Answer from the drawing. Dimensions are ordinates in mm from the lowest x, y and z of the part. A direction names the side the tool comes from. Round coordinates to 2 decimals unless told otherwise and drop trailing zeros. Order: outer loops, then holes, each group sorted by start corner. A loop starts at its lowest first (then second) coordinate and runs counter-clockwise, first axis right, second up. Notation, with made-up numbers: (54.5, 29.25) - (66.5, 29.25) arc R34 ccw to (66.5, 68.25) - close; hole circle Ø10 at (86, 47.5). An arc over 180 degrees is marked (long way). One line per question, with ' | ' between items. Start each with the question number.
1) For the marked faces 1 and 2, determine the directions among +Z, -Z, +X, -X, +Y, -Y from which every point of the face is accessible in a straight line to the end or side of a thin tool.
2) The part is cut by section D-D, the plane z = 1.35. Give the vertices of the cut face in (x, y).
3) Straight lines are drawn through the part: line 1 (Y direction, x = 6.5, z = 0.05); line 2 (Z direction, x = 4, y = 9.5); line 3 (Y direction, x = 5, z = 1.75) (1 decimal). For each, find the intervals that lie inside material, in ascending order. Write a range as from..to.
4) Flat-ended cylindrical pins translate along their axes: pin 1 (1 mm diameter, centred on y = 8, z = 2.5, fed in from +X); pin 2 (4 mm diameter, centred on x = 7.5, y = 8, fed in from -Z); pin 3 (2.5 mm diameter, centred on x = 7.5, y = 5, fed in from +Z); pin 4 (1 mm diameter, centred on y = 5, z = 4, fed in from -X). Find the tip coordinate at first contact, or state that the pin passes through.
5) The mould has two halves that part along X. Classify the marked faces 3, 4, 5 and 6: pulls with the +X half, pulls with the -X half, needs draft (parallel to the pull), parting line crosses it, or undercut.
6) The part is cut by section A-A, the plane z = 2.7. Give the vertices of the cut face in (x, y).
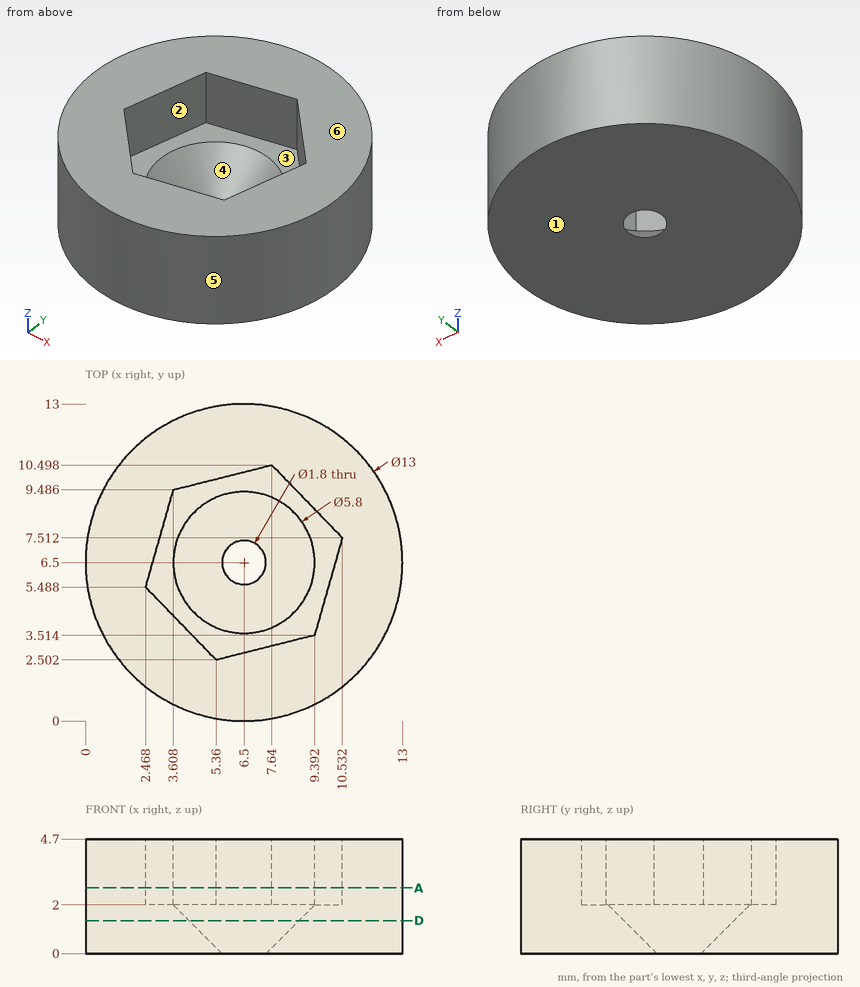
Values:
1) face 1: -Z, +X, -X, +Y, -Y | face 2: +Z
2) outline: circle Ø13 at (6.5, 6.5); hole circle Ø4.5 at (6.5, 6.5)
3) line 1: y = 0..5.55, 7.45..13 | line 2: z = 0..2 | line 3: y = 0.2..4.3, 8.7..12.8
4) pin 1: stops at x = 12.92 | pin 2: stops at z = 0 | pin 3: stops at z = 2 | pin 4: stops at x = 0.08
5) face 3: undercut | face 4: undercut | face 5: parting line crosses it | face 6: needs draft
6) outline: circle Ø13 at (6.5, 6.5); hole (2.47, 5.49) - (5.36, 2.5) - (9.39, 3.51) - (10.53, 7.51) - (7.64, 10.5) - (3.61, 9.49) - close
